Source: three-view drawing plus pictorial views. Frame: mm from the lowest corner of the part. Round coordinates to 2 decimals unless told otherwise and drop trailing zeros. Loops run counter-clockwise (first coordinate to the right, second up) from the corner with the lowest first, then second, coordinate; pieces in that order, holes last. Notation, with made-up numbers: (-11, 40.25) -> (24, 40.25) arc R20 ccw to (24, 62.25) -> close; hole circle Ø6 at (-38, 5.25). An arc over 180 degrees is marked (long way). One line per question, with ' | ' between items. Start each with the question number.
Q1. Material intervals for L1, parallel to Z at x = 31.75, y = 2.5; L2, parallel to X at y = 4.25, z = 10; L3, parallel to X at y = 7.25, z = 7.75, sorted ascending.
Q2. Cut plane B-B on y = 7.25. State how many separate pieces and enclosed holes the cut face has, and give its area (3 significant figures).
Q3. Mould query, pull axis Z, two halves, no side actions, for the marked faces 1, 2, 3 and 4. Classes: pulls with the +Z half, pulls with the -Z half, needs draft (parallel to the pull), parting line crosses it, or undercut.
Q4. Cut plane A-A on x = 31.75. Return loops of the section in (y, z).
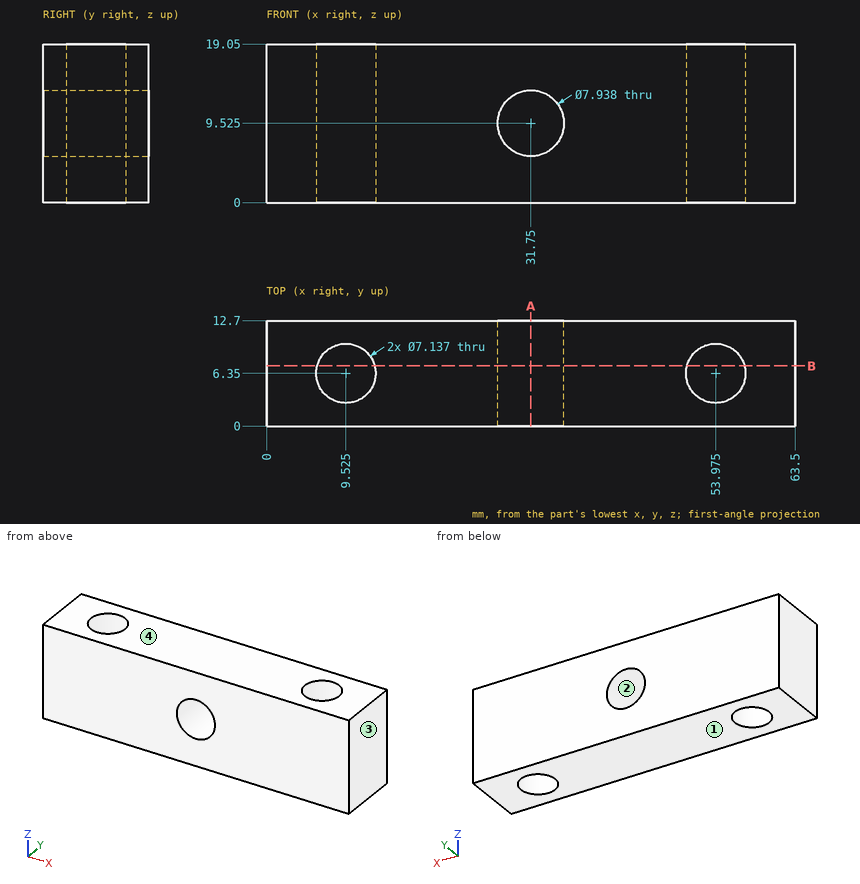
Results:
1) L1: 0 to 5.56, 13.49 to 19.05 | L2: 0 to 6.64, 12.41 to 27.81, 35.69 to 51.09, 56.86 to 63.5 | L3: 0 to 6.07, 12.98 to 28.2, 35.3 to 50.52, 57.43 to 63.5
2) separate pieces: 3 | enclosed holes: 1 | area: 897 mm^2
3) face 1: pulls with the -Z half | face 2: undercut | face 3: needs draft | face 4: pulls with the +Z half
4) outline: (0, 0) -> (12.7, 0) -> (12.7, 5.56) -> (0, 5.56) -> close; (0, 13.49) -> (12.7, 13.49) -> (12.7, 19.05) -> (0, 19.05) -> close
